Here's the drawing with two shaded views (mm, measured from the low corner). I have some questions. A direction names the side the tool comes from. Round coordinates to 2 decimals unless told otherwise and drop trailing zeros. Order: outer loops, then holes, each group sorted by start corner. A loop starts at its lowest first (then second) coordinate and runs counter-clockwise, first axis right, second up. Notation, with made-up numbers: (15, 68) -> (44, 68) arc R18 ccw to (44, 87) -> close; hole circle Ø3 at (25.5, 26). An arc over 180 degrees is marked (long way). Use a Markdown table: item, result. Add a question column.
Q1. We'd pull the mould along X, two halves only. Please class the marked faces 3, 4 and 5: +X half, -X half, draft (parallel to the pull), parting line (faces both ways), or undercut.
Q2. For the marked faces 1 and 2, which set-ups out of +Z, -Z, +X, -X, +Y, -Y let a thin tool reach every point of the face, with its end or its side?
Q3. I'm going to push flat-ended pins straight in: pin 1 Ø1 at (x, z) = (6, 7.5) entering from +Y; pin 2 Ø3 at (x, z) = (7, 3) entering from -Y. Where does each tip first touch, or does it pass through?
Q4. If we section it at C-C on x = 5: List the corners of the cut face in (y, z) for me.
Q5. If we section it at A-A on y = 7: List the corners of the cut face in (x, z) for me, plus the area to 3 significant figures.
Q6. I need wall thicknesses on line 1 along X through (y, z) = (7, 2.75); line 2 along X through (y, z) = (10.75, 8.75); line 3 along Y through (x, z) = (5, 2.5). Which ranges of each line are inside material? Lowest first, please. Write a range as [from, to].
Q7. If we section it at B-B on z = 10.5: List the corners of the cut face in (x, y) for me, plus the area to 3 significant figures.
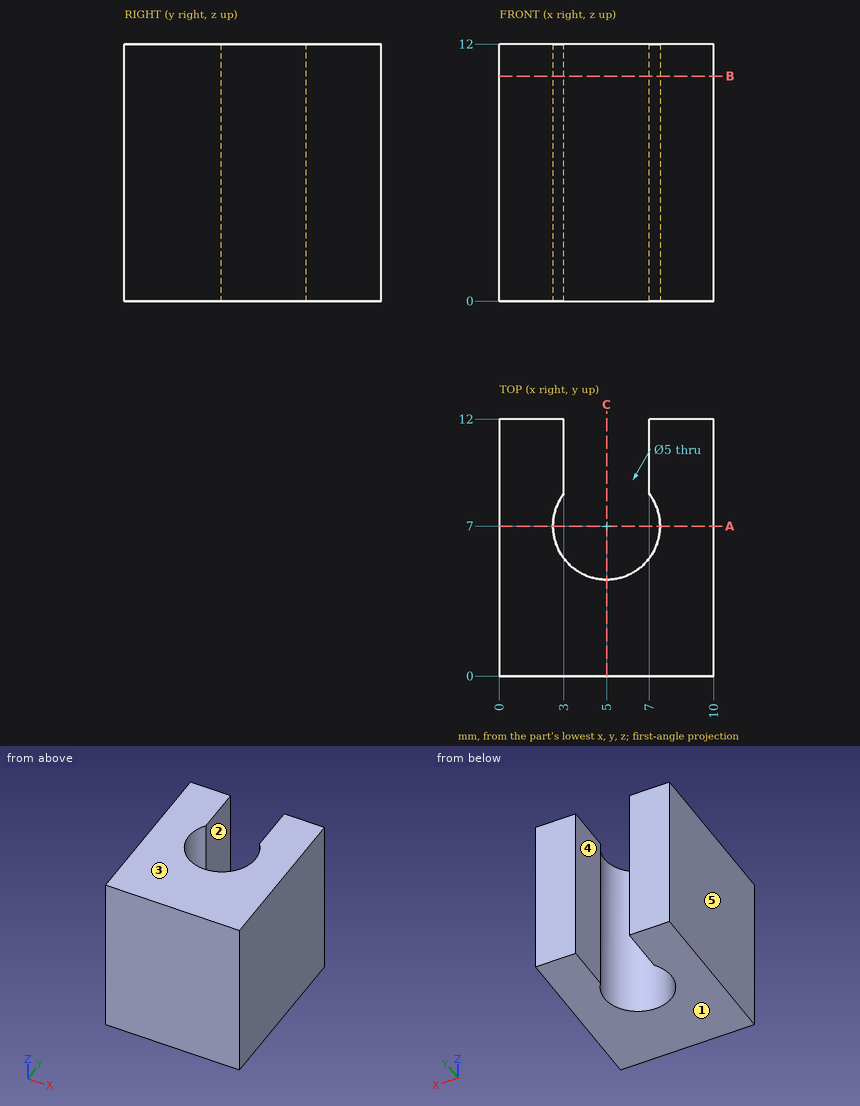
Answer below:
| question | item | result |
|---|---|---|
| 1 | face 3 | draft |
| 1 | face 4 | undercut |
| 1 | face 5 | -X half |
| 2 | face 1 | -Z, +X, -X, +Y, -Y |
| 2 | face 2 | +Z, -Z, +Y |
| 3 | pin 1 | y = 5 |
| 3 | pin 2 | y = 0 |
| 4 | outline | (0, 0) -> (4.5, 0) -> (4.5, 12) -> (0, 12) -> close |
| 5 | outline | (0, 0) -> (2.5, 0) -> (2.5, 12) -> (0, 12) -> close; (7.5, 0) -> (10, 0) -> (10, 12) -> (7.5, 12) -> close |
| 5 | area | 60.0 mm² |
| 6 | line 1 | [0, 2.5], [7.5, 10] |
| 6 | line 2 | [0, 3], [7, 10] |
| 6 | line 3 | [0, 4.5] |
| 7 | outline | (0, 0) -> (10, 0) -> (10, 12) -> (7, 12) -> (7, 8.5) arc R2.5 cw (long way) to (3, 8.5) -> (3, 12) -> (0, 12) -> close |
| 7 | area | 89.2 mm² |
